Can you work these out from the model? Positions are in its coordinate system, mm. Face numbers are marked on the shaded views. A direction names the side the tool comes from. Coordinates: 2 decimals unless noted, no trailing zeros. Write each loop counter-clockwise with the first axis right and the second up, starting at its lowest first coordinate (ties: lowest second). Pieces come first, ordered by that corner, then holes. Notation, with made-up numbers: (81.5, -9.5) - (88.5, -9.5) arc R20 cw to (88.5, 5.5) - close; hole circle Ø9 at (41.5, -20.5). An arc over 180 degrees is marked (long way). Use one line per item in the form item = value. Start each with the question number.
(1) If we section it at C-C on x = 22: Please give me the cut outline in (y, z), then the cut area to 3 significant figures.
(2) If we section it at A-A on z = 0: Please give me the cut outline in (x, y).
(3) On a 3-axis mill with a long thin cutter (end or side, diameter ignored), from which of +Z, -Z, +X, -X, +Y, -Y can I reach the whole of each face in a straight line? I mean the marked faces 1, 2 and 3. Say none if no direction works.
(4) For pin 1 Ø6 at (x, y) = (-6.5, 1) entering from +Z; pin 2 Ø6 at (x, y) = (4, -0.5) entering from -Z; pin 3 Ø12 at (y, z) = (0, 0) entering from -X; pin 4 Ø6 at (y, z) = (3.5, 7.5) entering from -X, each with a flat end and sliding along its axis, tell me the tip position at first contact or that it passes through.
(5) If we section it at B-B on y = 0: Please give me the cut outline in (x, z), then the cut area to 3 significant figures.
(6) Thinking about a two-plate mould opening in Z: for the marked faces 4, 5, 6 and 7, which applies, pulls with the +Z half, pulls with the -Z half, needs draft (parallel to the pull), parting line crosses it, or undercut?
(7) If I drill on probe 1 along Y at (x, z) = (0, -23); probe 2 along Z at (x, y) = (1, -1), over which ranges is the centre line in solid material (lowest first)? Write a range as from..to.
Autodesk Inventor part; units mm, degrees
ref_plane "YZ Plane" through (0, 0, 0) normal (1, 0, 0) x (0, 1, 0)
ref_plane "XZ Plane" through (0, 0, 0) normal (0, 1, 0) x (-1, 0, 0)
ref_plane "XY Plane" through (0, 0, 0) normal (0, 0, 1) x (1, 0, 0)
sketch "Sketch1" plane through (0, 0, 0) normal (1, 0, 0) x (0, 1, 0)
  line L0 (31.9501, 0) -> (-31.3732, 0)
  line L1 (0, 29.3537) -> (0, -50.8461) construction
  line L2 (25, 25) -> (-25, 25)
  line L3 (-25, 25) -> (-25, -25)
  line L4 (-25, -25) -> (25, -25)
  line L5 (25, -25) -> (25, 25)
  circle A0 centre (0.2885, 0) radius 10
  point P0 (0, 0)
  dimension "d0" = 50
  dimension "d1" = 50
  dimension "d3" = 50
  dimension "d4" = 50
  dimension "d5" = 20
sketch "Sketch2" plane through (0, 0, 0) normal (0, 0, 1) x (1, 0, 0)
  line L0 (0, 17.9809) -> (0, -21.5338)
  line L1 (-16.5078, 0) -> (19.6274, 0)
  line L2 (-25, 25) -> (25, 25)
  line L3 (25, 25) -> (25, -25)
  line L4 (25, -25) -> (-25, -25)
  line L5 (-25, -25) -> (-25, 25)
  circle A0 centre (0, 0) radius 10
  dimension "d6" = 50
  dimension "d7" = 50
  dimension "d8" = 25
  dimension "d9" = 50
  dimension "d10" = 20
extrude "Extrusion1" add sketch "Sketch2" along normal mid plane 50
extrude "Extrusion2" add sketch "Sketch2" along normal mid plane 30 contours A0 L1 L0 | L0 L1 A0 | L1 A0 L0 | L0 A0 L1
sketch "Sketch3" plane through (-25, -25, 25) normal (-1, 0, 0) x (0, 0, 1)
  circle A0 centre (-25, 25) radius 10
  dimension "d15" = 20
extrude "Extrusion3" cut sketch "Sketch3" against normal blind 10
sketch "Sketch4" plane through (25, -25, 25) normal (1, 0, 0) x (0, 0, -1)
  circle A0 centre (25, 25) radius 10
  dimension "d18" = 20
extrude "Extrusion4" cut sketch "Sketch4" against normal blind 10
properties part number "CT_02"
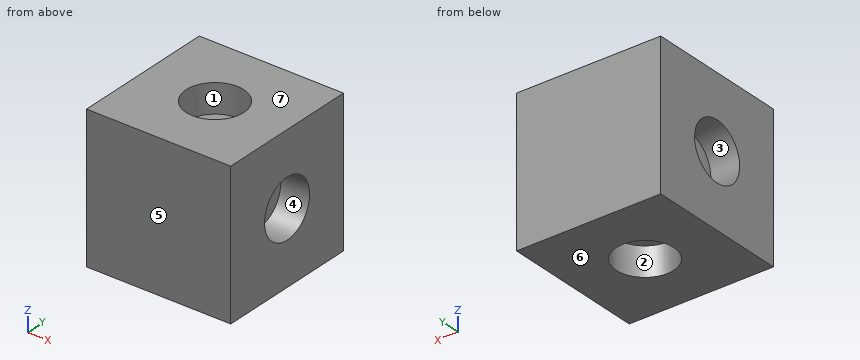
Reported:
q1.outline = (-25, -25) - (25, -25) - (25, 25) - (-25, 25) - close; hole circle Ø20 at (0, 0)
q1.area = 2,190 mm2
q2.outline = (-25, -25) - (25, -25) - (25, -10) - (15, -10) - (15, 10) - (25, 10) - (25, 25) - (-25, 25) - (-25, 10) - (-15, 10) - (-15, -10) - (-25, -10) - close
q3.face_1 = +Z
q3.face_2 = -Z
q3.face_3 = -X
q4.pin_1 = 15
q4.pin_2 = -15
q4.pin_3 = -15
q4.pin_4 = -25
q5.outline = (-25, -25) - (-10, -25) - (-10, -15) - (10, -15) - (10, -25) - (25, -25) - (25, -10) - (15, -10) - (15, 10) - (25, 10) - (25, 25) - (10, 25) - (10, 15) - (-10, 15) - (-10, 25) - (-25, 25) - (-25, 10) - (-15, 10) - (-15, -10) - (-25, -10) - close
q5.area = 1,700 mm2
q6.face_4 = undercut
q6.face_5 = needs draft
q6.face_6 = pulls with the -Z half
q6.face_7 = pulls with the +Z half
q7.probe_1 = -25..-10, 10..25
q7.probe_2 = -15..15
